Autodesk Inventor part; units mm, degrees
ref_plane "YZ Plane" through (0, 0, 0) normal (1, 0, 0) x (0, 1, 0)
ref_plane "XZ Plane" through (0, 0, 0) normal (0, 1, 0) x (-1, 0, 0)
ref_plane "XY Plane" through (0, 0, 0) normal (0, 0, 1) x (1, 0, 0)
sketch "Sketch1" plane through (0, 0, 0) normal (0, 1, 0) x (-1, 0, 0)
  line L0 (-22.6949, -27.051) -> (22.6949, -27.051)
  line L1 (22.6949, -27.051) -> (22.6949, 27.051)
  line L2 (22.6949, 27.051) -> (-22.6949, 27.051)
  line L3 (-22.6949, 27.051) -> (-22.6949, -27.051)
  line L4 (-22.6949, -27.051) -> (22.6949, 27.051) construction
  line L5 (22.6949, -27.051) -> (-22.6949, 27.051) construction
  point P0 (0, 0)
  dimension "d0" = 45.3898
  dimension "d1" = 54.102
extrude "Extrusion1" add sketch "Sketch1" along normal blind 2.54
sketch "Sketch2" plane through (0, 2.54, 0) normal (0, 1, 0) x (1, 0, 0)
  line L0 (-9.9949, 14.351) -> (3.6449, 14.351)
  line L1 (3.6449, 14.351) -> (3.6449, -14.351)
  line L2 (3.6449, -14.351) -> (-9.9949, -14.351)
  line L3 (-9.9949, -14.351) -> (-9.9949, 14.351)
  line L4 (22.6949, -27.051) -> (22.6949, 27.051)
  line L5 (22.6949, 27.051) -> (-22.6949, 27.051)
  point P0 (0, 0)
  dimension "d4" = 13.6398
  dimension "d5" = 28.702
  dimension "d6" = 19.05
  dimension "d7" = 12.7
extrude "Extrusion2" cut sketch "Sketch2" against normal through all
sketch "Sketch3" plane through (0, 2.54, 0) normal (0, 1, 0) x (1, 0, 0)
  circle A0 centre (17.2339, -5.588) radius 1.778
  line L0 (22.6949, -27.051) -> (22.6949, 27.051)
  circle A1 centre (17.2339, 5.588) radius 1.778
  circle A2 centre (17.2339, 13.4747) radius 1.778
  circle A3 centre (17.2339, -13.4747) radius 1.778
  line L1 (-22.6949, -27.051) -> (22.6949, -27.051)
  line L2 (22.6949, 27.051) -> (-22.6949, 27.051)
  point P0 (0, 0)
  dimension "d10" = 3.556
  dimension "d12" = 3.556
  dimension "d13" = 14.732
  dimension "d14" = 7.62
  dimension "d15" = 3.556
  dimension "d16" = 3.556
  dimension "d17" = 4.3307
  dimension "d18" = 4.3307
  dimension "d19" = 26.9494
  dimension "d20" = 13.5763
  dimension "d21" = 13.5763
extrude "Extrusion3" cut sketch "Sketch3" against normal through all
properties part number "switch holder"
The listing builds one solid part. Answer for the finished solid, in the listing's coordinates (mm). A direction names the side the tool comes from. Give positions to 0.01 mm unless a question says otherwise; leave off trailing zeros. Order: outer loops, then holes, each group sorted by start corner. A loop starts at its lowest first (then second) coordinate and runs counter-clockwise, first axis right, second up. Notation, with made-up numbers: (61.25, -38) -> (111.25, -38) arc R17 cw to (111.25, -33) -> close; hole circle Ø6 at (42.25, -28.75). An arc over 180 degrees is marked (long way). Answer as a JSON object with one key per item and string values. Group by question number.
Item 1: The part is cut by section A-A on x = 1. Write down the section's boundary in (y, z), and give its area (3 significant figures).
Item 2: A tool of negligible diameter and unlimited length cuts with its end or side. For faces 4 (the flat face through (22.695, 1, 0)), 5 (the flat face through (-9.995, 1, 0)), from which of +Z, -Z, +X, -X, +Y, -Y can it reach the whole face along a straight path? Write none if from no direction.
Item 3: Flat-ended cylindrical pins translate along their axes: pin 1 (3 mm diameter, centred on x = 17.23, z = 13.47, fed in from -Y); pin 2 (4 mm diameter, centred on x = 17.23, z = -13.47, fed in from +Y). Find the tip coordinate at first contact, or state that the pin passes through.
Item 4: Consider L1, parallel to X at y = 0.4, z = -3; L2, parallel to X at y = 0.3, z = 6.5; L3, parallel to Z at x = 3, y = 1.4. Determine where each line is inside the solid, lowest interval first. Write a range as from..to.
Item 5: Determine the mould class of faces 1 (the flat face through (-3, 1, -14.351)), 2 (the flat face through (0, 1, -27.051)), 3 (the flat face through (-22.695, 1, 0)) for opening direction Z: pulls with the +Z half, pulls with the -Z half, needs draft (parallel to the pull), parting line crosses it, or undercut.
Item 6: The part is cut by section B-B on x = 16.5. Write down the section's boundary in (y, z), and give its area (3 significant figures).
Item 7: The part is cut by section C-C on y = 1. Write down the section's boundary in (x, z), and give its area (3 significant figures).
Result set:
{
 "1": {"outline": "(0, -27.05) -> (2.54, -27.05) -> (2.54, -14.35) -> (0, -14.35) -> close; (0, 14.35) -> (2.54, 14.35) -> (2.54, 27.05) -> (0, 27.05) -> close", "area": "64.5 mm²"},
 "2": {"face 4": "+Z, -Z, +X, +Y, -Y", "face 5": "+Y, -Y"},
 "3": {"pin 1": "through", "pin 2": "y = 2.54"},
 "4": {"L1": "-22.69..-9.99, 3.64..22.69", "L2": "-22.69..-9.99, 3.64..15.71, 18.76..22.69", "L3": "-27.05..-14.35, 14.35..27.05"},
 "5": {"face 1": "undercut", "face 2": "pulls with the -Z half", "face 3": "needs draft"},
 "6": {"outline": "(0, -27.05) -> (2.54, -27.05) -> (2.54, -15.09) -> (0, -15.09) -> close; (0, -11.86) -> (2.54, -11.86) -> (2.54, -7.21) -> (0, -7.21) -> close; (0, -3.97) -> (2.54, -3.97) -> (2.54, 3.97) -> (0, 3.97) -> close; (0, 7.21) -> (2.54, 7.21) -> (2.54, 11.86) -> (0, 11.86) -> close; (0, 15.09) -> (2.54, 15.09) -> (2.54, 27.05) -> (0, 27.05) -> close", "area": "105 mm²"},
 "7": {"outline": "(-22.69, -27.05) -> (22.69, -27.05) -> (22.69, 27.05) -> (-22.69, 27.05) -> close; hole (-9.99, -14.35) -> (3.64, -14.35) -> (3.64, 14.35) -> (-9.99, 14.35) -> close; hole circle Ø3.56 at (17.23, -13.47); hole circle Ø3.56 at (17.23, -5.59); hole circle Ø3.56 at (17.23, 5.59); hole circle Ø3.56 at (17.23, 13.47)", "area": "2,020 mm²"}
}
